Could you check a few things on this model? Use its own coordinates, in mm. Face numbers are marked on the shaded views. A direction names the side the tool comes from. Coordinates: 2 decimals unless noted, no trailing zeros. Loops run counter-clockwise (first coordinate to the right, second up) from the corner with the lowest first, then second, coordinate; pieces in that order, holes last. Notation, with made-up numbers: M 18,26 L 46,26 A22 cw 46,58 Z; hole C -12.75,4.25 d7. An arc over 180 degrees is marked long. Write each question's results on one line, items separated by ' | '.
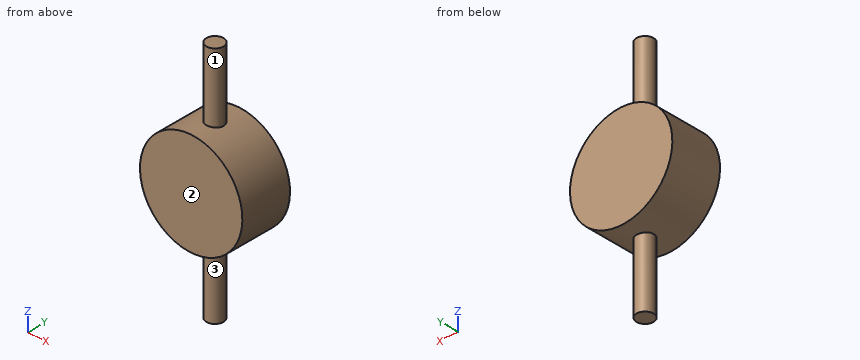
```python
from build123d import *

# Parameters (mm, degrees)
SKETCH1_R                = 15
BOSS_EXTRUDE1_DEPTH      = 15
BOSS_EXTRUDE2_DEPTH      = 35
BOSS_EXTRUDE2_DEPTH_BACK = 35
SKETCH2_R                = 2.5


with BuildPart() as part:
    # Sketch1 → Boss-Extrude1 (new body)
    with BuildSketch(Plane(origin=(0, 0, 0), x_dir=(1, 0, 0), z_dir=(0, 1, 0))):
        with Locations(Location((0, 0, 0), (0, 0, 270))):
            Circle(SKETCH1_R)
    extrude(amount=BOSS_EXTRUDE1_DEPTH)

    # Sketch2 → Boss-Extrude2 (add, two sides: drawn at the far end of the back side and taken through both)
    with BuildSketch(Plane.XY.offset(-BOSS_EXTRUDE2_DEPTH_BACK)):
        with Locations((0, 7.484573098)):
            Circle(SKETCH2_R)
    extrude(amount=BOSS_EXTRUDE2_DEPTH + BOSS_EXTRUDE2_DEPTH_BACK)


solid = part.part
```
(1) Imagine slicing it at B-B, the plane y = 8.5. List the corners of the cut face in (x, z) for me.
Reported:
outline: M -2.28,-35 L 2.28,-35 L 2.28,-14.83 A15 ccw 2.28,14.83 L 2.28,35 L -2.28,35 L -2.28,14.83 A15 ccw -2.28,-14.83 Z
(2) Imagine slicing it at A-A, the plane x = 0. List the corners of the cut face in (y, z) for me, and give its area (3 significant figures).
Reported:
outline: M 0,-15 L 4.98,-15 L 4.98,-35 L 9.98,-35 L 9.98,-15 L 15,-15 L 15,15 L 9.98,15 L 9.98,35 L 4.98,35 L 4.98,15 L 0,15 Z | area: 650 mm2
(3) Imagine slicing it at C-C, the plane z = -26. List the corners of the cut face in (x, y) for me.
Reported:
outline: C 0,7.48 d5
(4) Will these pins go through, and if not, where does the flat tip stop? P1, Ø8, axis at x = 3, z = -25.5, coming from the -Y side; P2, Ø5, axis at y = 4, z = 9.5, coming from the -X side; P3, Ø1.5, axis at x = -6, y = 10.5, coming from the +Z side.
Reported:
P1: stops at y = 4.98 | P2: stops at x = -13.27 | P3: stops at z = 14.05
(5) Which directions (+Z, -Z, +X, -X, +Y, -Y) give clear straight access to the entire face, cutting with the end or side of a thin tool? Please do the marked faces 1, 2 and 3.
Reported:
face 1: +Z | face 2: +Z, -Z, +X, -X, -Y | face 3: -Z
(6) Imagine slicing it at D-D, the plane y = 3. List the corners of the cut face in (x, z) for me.
Reported:
outline: C 0,0 d30
(7) Please list where these lines run through material, in increasing order: probe 1 along X at (y, z) = (6.5, 0); probe 2 along Y at (x, z) = (0, 26.5); probe 3 along Z at (x, y) = (2, 14). Write a range as from..to.
Reported:
probe 1: x = -15..15 | probe 2: y = 4.98..9.98 | probe 3: z = -14.87..14.87
